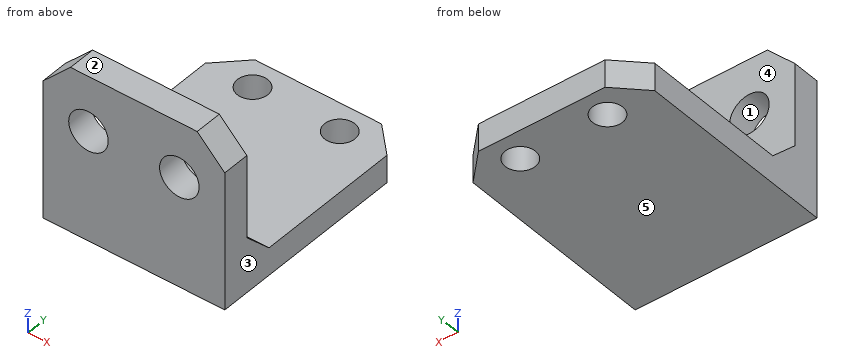
from build123d import *

# Parameters (mm, degrees)
SKETCH1_W           = 19.8
SKETCH1_H           = 25
SKETCH1_R           = 1.65
BOSS_EXTRUDE1_DEPTH = 3
SKETCH2_W           = 19.8
SKETCH2_H           = 3
BOSS_EXTRUDE2_DEPTH = 15
CHAMFER1_SIZE       = 3
SKETCH4_R           = 2.15
CUT_EXTRUDE1_DEPTH  = 15
CHAMFER2_SIZE       = 3


with BuildPart() as part:
    # Sketch1 → Boss-Extrude1 (new body)
    with BuildSketch(Plane.XY):
        with Locations((0, 1.287671233)):
            Rectangle(SKETCH1_W, SKETCH1_H)
        with Locations((-4.75, 10.787671233)):
            Circle(SKETCH1_R, mode=Mode.SUBTRACT)
        with Locations(Location((4.75, 10.787671233, 0), (0, 0, 180))):
            Circle(SKETCH1_R, mode=Mode.SUBTRACT)
    extrude(amount=BOSS_EXTRUDE1_DEPTH)

    # Sketch2 → Boss-Extrude2 (add)
    with BuildSketch(Plane.XY.offset(3)):
        with Locations((0, -9.712328767)):
            Rectangle(SKETCH2_W, SKETCH2_H)
    extrude(amount=BOSS_EXTRUDE2_DEPTH)

    # Chamfer1
    chamfer1_edges = [part.edges().sort_by_distance(p)[0] for p in [
        (0, -8.212328767, 3),
        (-9.9, 13.787671233, 1.5),
        (9.9, 13.787671233, 1.5),
    ]]
    chamfer(chamfer1_edges, length=CHAMFER1_SIZE)

    # Sketch4 → Cut-Extrude1 (cut)
    with BuildSketch(Plane(origin=(0, -8.212328767, 0), x_dir=(1, 0, 0), z_dir=(0, 1, 0))):
        with Locations(Location((4.95, -12, 0), (0, 0, 270))):
            Circle(SKETCH4_R)
        with Locations(Location((-4.95, -12, 0), (0, 0, 180))):
            Circle(SKETCH4_R)
    extrude(amount=-CUT_EXTRUDE1_DEPTH, mode=Mode.SUBTRACT)

    # Chamfer2
    chamfer2_edges = [part.edges().sort_by_distance(p)[0] for p in [
        (-9.9, -9.712328767, 18),
        (9.9, -9.712328767, 18),
    ]]
    chamfer(chamfer2_edges, length=CHAMFER2_SIZE)


solid = part.part
Geometry check sheet. Reference: the model listing, model coordinates, mm. Face numbers are marked on the shaded views. A direction names the side the tool comes from. Give positions to 0.01 mm unless a question says otherwise; leave off trailing zeros. Loops run counter-clockwise (first coordinate to the right, second up) from the corner with the lowest first, then second, coordinate; pieces in that order, holes last. Notation, with made-up numbers: M 68,5 L 81,5 A11 cw 81,14 Z; hole C 15.5,54 d11. An arc over 180 degrees is marked long. Answer as a JSON object with one key per item and string values. Group by question number.
Item 1: Sectioned sample at D-D on x = -2.25. Record the boundary of the cut face in (y, z), plus the area to 4 significant figures.
Item 2: Sectioned sample at C-C on x = 5.75. Record the boundary of the cut face in (y, z), plus the area to 3 significant figures.
Item 3: Material ranges on L1, parallel to Y at x = 4.75, z = 0.75; L2, parallel to Z at x = -4.95, y = -8.9; L3, parallel to Z at x = 0.5, y = 2, recorded low to high.
Item 4: Sectioned sample at B-B on z = 2.5. Record the boundary of the cut face in (x, y).
Item 5: Access from +Z, -Z, +X, -X, +Y, -Y to the whole of each face (thin tool, end or side, straight path). Record for the marked faces 4 and 5.
Item 6: Gauge pin test, flat ends, axial feed: pin 1 (5.5 mm diameter, centred on x = 4.75, y = 10.79, fed in from -Z); pin 2 (5 mm diameter, centred on x = -2.5, y = 7, fed in from +Z); pin 3 (3.5 mm diameter, centred on x = -4.5, z = 11, fed in from +Y). Record the tip position at first contact, or that the pin passes through.
Item 7: Mould release check, pull along Z, two halves, no side actions. Record for the marked faces 1, 2 and 3: pulls with the +Z half, pulls with the -Z half, needs draft (parallel to the pull), parting line crosses it, or undercut.
Item 8: Sectioned sample at A-A on z = 12. Record the boundary of the cut face in (x, y).
Findings below:
{
 "1": {"outline": "M -11.21,0 L 13.79,0 L 13.79,3 L -5.21,3 L -8.21,6 L -8.21,18 L -11.21,18 Z", "area": "124.5 mm2"},
 "2": {"outline": "M -11.21,0 L 9.48,0 L 9.48,3 L -5.21,3 L -8.21,6 L -8.21,10 L -11.21,10 Z; M -11.21,14 L -8.21,14 L -8.21,18 L -11.21,18 Z; M 12.1,0 L 13.79,0 L 13.79,3 L 12.1,3 Z", "area": "105 mm2"},
 "3": {"L1": "-11.21 to 9.14, 12.44 to 13.79", "L2": "0 to 9.85, 14.15 to 18", "L3": "0 to 3"},
 "4": {"outline": "M -9.9,-11.21 L 9.9,-11.21 L 9.9,10.79 L 6.9,13.79 L -6.9,13.79 L -9.9,10.79 Z; hole C -4.75,10.79 d3.3; hole C 4.75,10.79 d3.3"},
 "5": {"face 4": "+Z, +X, -X, +Y", "face 5": "-Z, +X, -X, +Y, -Y"},
 "6": {"pin 1": "z = 0", "pin 2": "z = 3", "pin 3": "y = -8.21"},
 "7": {"face 1": "undercut", "face 2": "pulls with the +Z half", "face 3": "needs draft"},
 "8": {"outline": "M -9.9,-11.21 L -7.1,-11.21 L -7.1,-8.21 L -9.9,-8.21 Z; M -2.8,-11.21 L 2.8,-11.21 L 2.8,-8.21 L -2.8,-8.21 Z; M 7.1,-11.21 L 9.9,-11.21 L 9.9,-8.21 L 7.1,-8.21 Z"}
}
